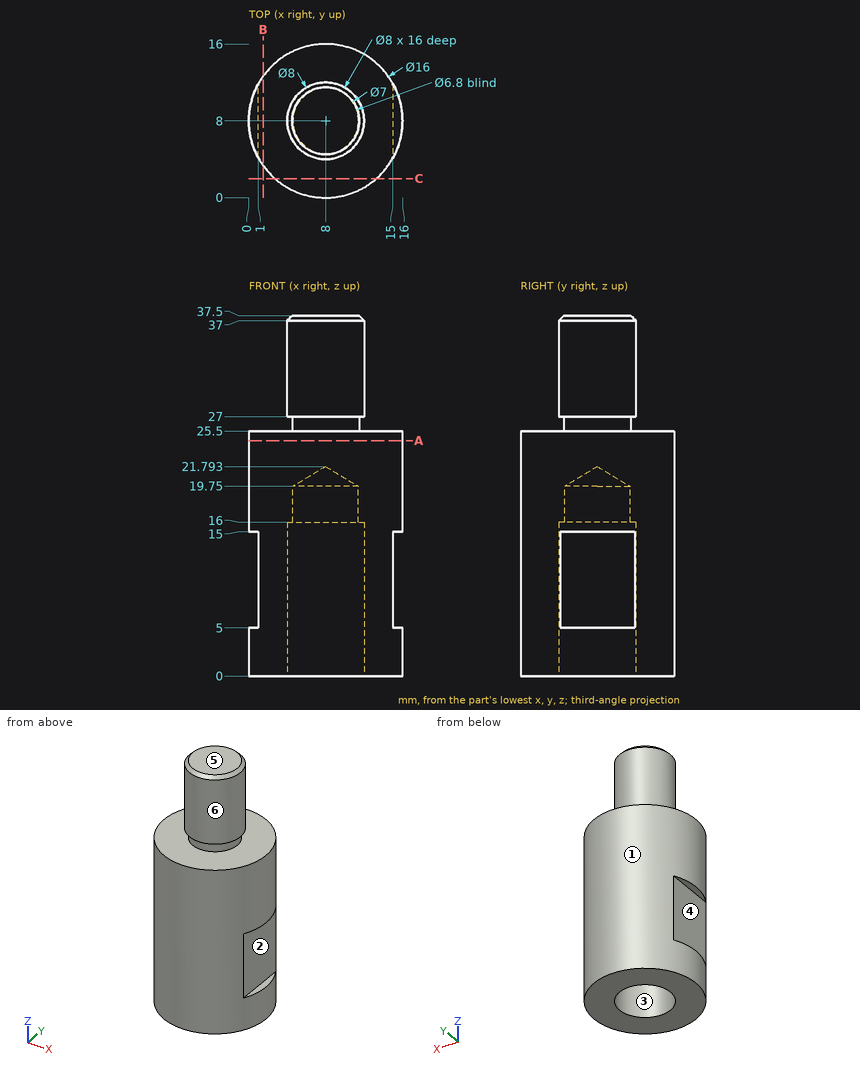
Print and shaded views of the part. All mm, measured from the part's lowest x, y and z. A direction names the side the tool comes from. Round coordinates to 2 decimals unless told otherwise and drop trailing zeros. Write each loop counter-clockwise with the first axis right and the second up, starting at its lowest first coordinate (ties: lowest second). Pieces come first, ordered by that corner, then holes.
(1) 3-axis set-ups, long thin cutter, end or side, ignore diameter. For the marked faces 4, 5 and 6: which of +Z, -Z, +X, -X, +Y, -Y reach the whole face in a straight line?
(2) Slice it at C-C, the plane y = 2. Write the cut outline in (x, z).
(3) Drop flat-ended pins along their axis: P1, Ø9, axis at x = 8, y = 8, coming from the -Z side; P2, Ø1, axis at x = 10, z = 17.5, coming from the -Y side; P3, Ø0.8, axis at x = 0.5, y = 6.5, coming from the +Z side; P4, Ø6, axis at y = 6, z = 9, coming from the +X side. Give the stop position or say it passes through.
(4) Probe line 1 along Y through (x, z) = (8, 5); line 2 along Z through (x, y) = (4.5, 11); line 3 along Y through (x, z) = (8, 18.75). List the from-to ranges inside material, lowest first.
(5) Mould opens along Y. For the marked faces 1, 2 and 3 say: pulls with the +Y half, pulls with the -Y half, needs draft (parallel to the pull), parting line crosses it, or undercut.
(6) Slice it at A-A, the plane z = 24.5. Write the cut outline in (x, y).
(7) Slice it at B-B, the plane x = 1.5. Write the cut outline in (y, z).
From the geometry:
1. face 4: -X, +Y, -Y
1. face 5: +Z, +X, -X, +Y, -Y
1. face 6: +Z
2. outline: (2.71, 0) - (13.29, 0) - (13.29, 25.5) - (2.71, 25.5) - close
3. P1: stops at z = 0
3. P2: stops at y = 0.14
3. P3: stops at z = 25.5
3. P4: stops at x = 15
4. line 1: y = 0 to 4, 12 to 16
4. line 2: z = 0 to 25.5
4. line 3: y = 0 to 4.6, 11.4 to 16
5. face 1: parting line crosses it
5. face 2: needs draft
5. face 3: undercut
6. outline: circle Ø16 at (8, 8)
7. outline: (3.34, 0) - (12.66, 0) - (12.66, 25.5) - (3.34, 25.5) - close
